```python
from build123d import *

# Parameters (mm, degrees)
SKETCH1_R           = 0.75
BOSS_EXTRUDE1_DEPTH = 3


with BuildPart() as part:
    # Sketch1 → Boss-Extrude1 (new body)
    with BuildSketch(Plane.XY):
        Polygon((-15, 42.25), (-10, 42.25), (-10, 45.25), (-3.75, 45.25), (-3.75, 42.25), (3.75, 42.25), (3.75, 45.25), (10, 45.25), (10, 42.25), (15, 42.25), (15, -42.25), (10, -42.25), (10, -45.25), (3.75, -45.25), (3.75, -42.25), (-3.75, -42.25), (-3.75, -45.25), (-10, -45.25), (-10, -42.25), (-15, -42.25), align=None)
        with Locations((0, 29.5)):
            Circle(SKETCH1_R, mode=Mode.SUBTRACT)
        with Locations((7.5, 22)):
            Circle(SKETCH1_R, mode=Mode.SUBTRACT)
        with Locations((0, 14.5)):
            Circle(SKETCH1_R, mode=Mode.SUBTRACT)
        with Locations((-7.5, 22)):
            Circle(SKETCH1_R, mode=Mode.SUBTRACT)
        with Locations((0, 7.5)):
            Circle(SKETCH1_R, mode=Mode.SUBTRACT)
        with Locations((-7.5, 0)):
            Circle(SKETCH1_R, mode=Mode.SUBTRACT)
        with Locations((0, -7.5)):
            Circle(SKETCH1_R, mode=Mode.SUBTRACT)
        with Locations((7.5, 0)):
            Circle(SKETCH1_R, mode=Mode.SUBTRACT)
        with Locations((0, -14.5)):
            Circle(SKETCH1_R, mode=Mode.SUBTRACT)
        with Locations((-7.5, -22)):
            Circle(SKETCH1_R, mode=Mode.SUBTRACT)
        with Locations((0, -29.5)):
            Circle(SKETCH1_R, mode=Mode.SUBTRACT)
        with Locations((7.5, -22)):
            Circle(SKETCH1_R, mode=Mode.SUBTRACT)
    extrude(amount=BOSS_EXTRUDE1_DEPTH)


solid = part.part
```
Model file for the job. Use its own axes, mm. A direction names the side the tool comes from. Coordinates: 2 decimals unless noted, no trailing zeros. Loops run counter-clockwise (first coordinate to the right, second up) from the corner with the lowest first, then second, coordinate; pieces in that order, holes last. Notation, with made-up numbers: (11, -26) -> (54, -26) arc R25 cw to (54, -6) -> close; hole circle Ø5 at (28.25, 85.5). An arc over 180 degrees is marked (long way). Answer as a JSON object with one key per item and string values.
Q1. Pull direction Y, two halves, no side cores. Call faces 6 (the cylindrical face through (-7.663, 21.268, 1.479)), 7 (the flat face through (7, -45.25, 1)), 8 (the cylindrical face through (-0.163, -8.232, 1.479)), 9 (the flat face through (-15, -1, 1)): released by +Y, released by -Y, zero draft, split by the parting line, or undercut.
Report:
{"face 6": "undercut", "face 7": "released by -Y", "face 8": "undercut", "face 9": "zero draft"}
Q2. 3-axis set-ups, long thin cutter, end or side, ignore diameter. For faces 1 (the flat face through (10, -44, 1)), 2 (the flat face through (0, -42.25, 1)), 3 (the cylindrical face through (-0.098, -13.756, 1.479)), 4 (the flat face through (10, 44, 1)), 5 (the flat face through (0, 42.25, 1)): which of +Z, -Z, +X, -X, +Y, -Y reach the whole face in a straight line?
Report:
{"face 1": "+Z, -Z, +X, -Y", "face 2": "+Z, -Z, -Y", "face 3": "+Z, -Z", "face 4": "+Z, -Z, +X, +Y", "face 5": "+Z, -Z, +Y"}
Q3. Cut at B-B (x = -2.5). List the corners of the cut face in (y, z).
Report:
{"outline": "(-42.25, 0) -> (42.25, 0) -> (42.25, 3) -> (-42.25, 3) -> close"}
Q4. Cut at A-A (z = 1.4). State how many separate pieces and enclosed holes the cut face has, and give its area (3 significant figures).
Report:
{"separate pieces": "1", "enclosed holes": "12", "area": "2,590 mm2"}
Q5. Probe probe 1 along Y at (x, z) = (7.5, 0.15); probe 2 along Y at (x, z) = (8, 1.1); probe 3 along Y at (x, z) = (12.25, 0.3). List the from-to ranges inside material, lowest first.
Report:
{"probe 1": "y = -45.25 to -22.75, -21.25 to -0.75, 0.75 to 21.25, 22.75 to 45.25", "probe 2": "y = -45.25 to -22.56, -21.44 to -0.56, 0.56 to 21.44, 22.56 to 45.25", "probe 3": "y = -42.25 to 42.25"}
Q6. Flat gauge pins, fed straight in: P1, Ø1.5, axis at y = -44, z = 1.5, coming from the +X side; P2, Ø1.5, axis at x = -13, z = 1.5, coming from the -Y side; P3, Ø1.5, axis at y = 44, z = 1, coming from the -X side; P4, Ø0.9, axis at x = 0, y = 14.5, coming from the +Z side. Where does each tip first touch, or does it go through?
Report:
{"P1": "stops at x = 10", "P2": "stops at y = -42.25", "P3": "stops at x = -10", "P4": "passes through"}
